Part model, mm, in its own coordinate system. Face numbers are marked on the shaded views. Round coordinates to 2 decimals unless told otherwise and drop trailing zeros. Order: outer loops, then holes, each group sorted by start corner. A loop starts at its lowest first (then second) coordinate and runs counter-clockwise, first axis right, second up. Notation, with made-up numbers: M 29,83.25 L 75,83.25 A11 ccw 75,100.25 Z; hole C -5.5,51.25 d3. An arc over 180 degrees is marked long. Write each question's results on one line, items separated by ' | '. Start each with the question number.
1. Band-saw the part on A-A, the plane z = 74. List the corners of the cut face in (x, y).
2. Drop flat-ended pins along their axis: pin 1 Ø10 at (x, z) = (37.5, 65.5) entering from -Y; pin 2 Ø2.5 at (x, z) = (47.5, 2.5) entering from -Y; pin 3 Ø1 at (x, y) = (68.5, 32.5) entering from +Z. Give the stop position or say it passes through.
3. Probe L1, parallel to Y at x = 95, z = 31; L2, parallel to Y at x = 47, z = 8; L3, parallel to Z at x = 10.5, y = 33. List the from-to ranges inside material, lowest first. Write a range as [from, to].
4. Two-plate mould, pull along X, no slides. Class the marked faces 1, 2, 3 and 4: +X half, -X half, draft (parallel to the pull), parting line (faces both ways), or undercut.
5. Band-saw the part on B-B, the plane x = 82.5. List the corners of the cut face in (y, z) (3 decimals), then the cut area to 3 significant figures.
```python
from build123d import *

# Parameters (mm, degrees)
SKETCH1_W           = 111.76
SKETCH1_H           = 264.16
BOSS_EXTRUDE1_DEPTH = 104.77499999999999
SKETCH2_W           = 111.76
SKETCH2_H           = 38.1
CUT_EXTRUDE1_DEPTH  = 81.66099999999999
CUT_LOFT3_START     = -22
CUT_LOFT3_OUTLINE_W = 111.76
CUT_LOFT3_OUTLINE_H = 41.526476030000005
CUT_LOFT3_DEPTH     = 15.94808629
SKETCH7_W           = 109.22000000000003
SKETCH7_H           = 3.7934503700089675
CUT_EXTRUDE3_DEPTH  = 306.36634363498547
SKETCH8_RX          = 32.28826667150602
SKETCH8_RY          = 15.237159552845547
CUT_EXTRUDE4_DEPTH  = 2.54
SKETCH9_R           = 5.040527571520393
BOSS_EXTRUDE2_DEPTH = 6.35
SKETCH10_R          = 2.398168465987588
BOSS_EXTRUDE3_DEPTH = 2.54
FILLET1_R           = 6.35
FILLET2_R           = 1.27


with BuildPart() as part:
    # Sketch1 → Boss-Extrude1 (new body)
    with BuildSketch(Plane.XY):
        with Locations((55.88, 132.08)):
            Rectangle(SKETCH1_W, SKETCH1_H)
    extrude(amount=BOSS_EXTRUDE1_DEPTH)

    # Sketch2 → Cut-Extrude1 (cut)
    with BuildSketch(Plane.XY.offset(104.77499999999999)):
        with Locations((55.88, 19.05)):
            Rectangle(SKETCH2_W, SKETCH2_H)
    extrude(amount=-CUT_EXTRUDE1_DEPTH, mode=Mode.SUBTRACT)

    # Cut-Loft3: read off the stored shape, not the designer's step
    # Cut-Loft3 outline → Cut-Loft3 (cut)
    with BuildSketch(Plane(origin=(0, 0, 0), x_dir=(1, 0, 0), z_dir=(0, 0.3977658725333551, -0.9174869539387353)).offset(CUT_LOFT3_START)):
        with Locations((55.88, -23.386975308)):
            Rectangle(CUT_LOFT3_OUTLINE_W, CUT_LOFT3_OUTLINE_H)
    extrude(amount=CUT_LOFT3_DEPTH, mode=Mode.SUBTRACT)

    # Sketch7 → Cut-Extrude3 (cut, through all)
    with BuildSketch(Plane(origin=(0, 0, 0), x_dir=(-1, 0, 0), z_dir=(0, 0, -1))):
        with Locations((-55.88000000000001, 1.8967251850044837)):
            Rectangle(SKETCH7_W, SKETCH7_H)
    extrude(amount=-CUT_EXTRUDE3_DEPTH, mode=Mode.SUBTRACT)

    # Sketch8 → Cut-Extrude4 (cut)
    with BuildSketch(Plane.XY.offset(104.77499999999999)):
        with Locations(Location((55.88, 153.6634760331982), (0, 0, 90))):
            Ellipse(SKETCH8_RX, SKETCH8_RY)
    extrude(amount=-CUT_EXTRUDE4_DEPTH, mode=Mode.SUBTRACT)

    # Sketch9 → Boss-Extrude2 (add)
    with BuildSketch(Plane.XZ.offset(-38.1)):
        with Locations(Location((55.88, 64.40266714831378, 0), (0, 0, 90))):
            Circle(SKETCH9_R)
    extrude(amount=BOSS_EXTRUDE2_DEPTH)

    # Sketch10 → Boss-Extrude3 (add)
    with BuildSketch(Plane.XZ.offset(-31.75)):
        with Locations(Location((55.88, 64.40266714831378, 0), (0, 0, 270))):
            Circle(SKETCH10_R)
    extrude(amount=BOSS_EXTRUDE3_DEPTH)

    # Fillet1
    fillet1_edges = [part.edges().sort_by_distance(p)[0] for p in [
        (55.88, 264.16, 104.77499999999999),
        (55.88, 38.1, 104.77499999999999),
    ]]
    fillet(fillet1_edges, radius=FILLET1_R)

    # Fillet2
    fillet2_edges = [part.edges().sort_by_distance(p)[0] for p in [
        (0, 264.16, 49.2125),
        (0, 262.3001280605346, 102.91512806053457),
        (0, 38.1, 60.7695),
        (0, 39.959871939465415, 102.91512806053457),
        (111.76, 38.1, 60.7695),
        (111.76, 39.959871939465415, 102.91512806053457),
        (111.76, 264.16, 49.2125),
        (111.76, 262.3001280605346, 102.91512806053457),
        (0, 19.049999999822614, 14.855092514590622),
        (111.76, 19.04999999982261, 14.85509251459062),
        (0, 151.13, 104.77499999999999),
        (111.76, 151.13, 104.77499999999999),
    ]]
    fillet(fillet2_edges, radius=FILLET2_R)


solid = part.part
```
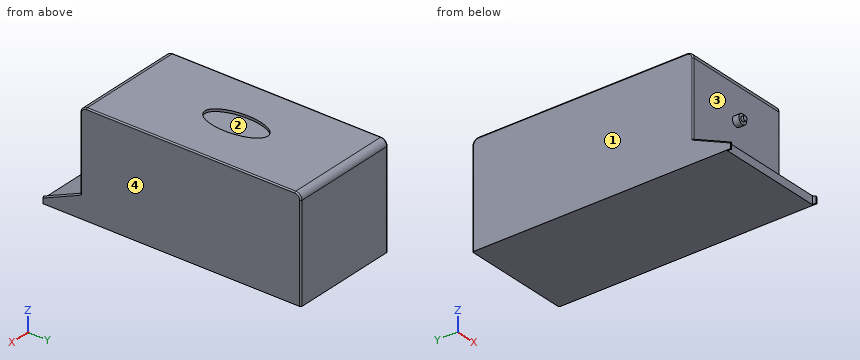
Solution:
1) outline: M 0,39.37 A1.27 ccw 1.27,38.1 L 110.49,38.1 A1.27 ccw 111.76,39.37 L 111.76,262.89 A1.27 ccw 110.49,264.16 L 1.27,264.16 A1.27 ccw 0,262.89 Z
2) pin 1: y = 38.1 | pin 2: y = 3.79 | pin 3: z = 20.9
3) L1: [38.1, 264.16] | L2: [3.79, 264.16] | L3: [0, 20.9]
4) face 1: -X half | face 2: undercut | face 3: draft | face 4: +X half
5) outline: M 3.793,0 L 264.16,0 L 264.16,98.425 A6.35 ccw 257.81,104.775 L 44.45,104.775 A6.35 ccw 38.1,98.425 L 38.1,23.114 L 3.793,8.241 Z | area: 24,200 mm^2
